```python
from build123d import *

# Parameters (mm, degrees)
SKETCH1_W           = 20
SKETCH1_H           = 30
BOSS_EXTRUDE1_DEPTH = 10
BOSS_EXTRUDE2_DEPTH = 10
SKETCH4_R           = 8.55
BOSS_EXTRUDE3_DEPTH = 10
FILLET1_R           = 5
BOSS_EXTRUDE4_DEPTH = 10
SKETCH6_R           = 1.25
CUT_EXTRUDE1_DEPTH  = 10


with BuildPart() as part:
    # Sketch1 → Boss-Extrude1 (new body)
    with BuildSketch(Plane(origin=(0, 0, 0), x_dir=(1, 0, 0), z_dir=(0, 1, 0))):
        with Locations((10, -15)):
            Rectangle(SKETCH1_W, SKETCH1_H)
    extrude(amount=BOSS_EXTRUDE1_DEPTH)

    # Sketch2 → Boss-Extrude2 (add)
    with BuildSketch(Plane(origin=(0, 10, 0), x_dir=(1, 0, 0), z_dir=(0, 1, 0))):
        Polygon((0, 0), (0, -10), (10, -10), (10, -30), (20, -30), (20, 0), align=None)
    extrude(amount=BOSS_EXTRUDE2_DEPTH)

    # Sketch4 → Boss-Extrude3 (add)
    with BuildSketch(Plane(origin=(0, 10, 0), x_dir=(1, 0, 0), z_dir=(0, 1, 0))):
        with BuildLine():
            Line((0, 0), (-17.51372228, 3.319944561))
            ThreePointArc((-17.51372228, 3.319944561), (-33.173842605, -6.829452566), (-23.846362973, -22.992612973))
            Line((-23.846362973, -22.992612973), (0, -30))
            Line((0, -30), (0, 0))
        make_face()
        with Locations(Location((-20, -10, 0), (0, 0, 270))):
            Circle(SKETCH4_R, mode=Mode.SUBTRACT)
    extrude(amount=-BOSS_EXTRUDE3_DEPTH)

    # Fillet1
    fillet1_edges = [part.edges().sort_by_distance(p)[0] for p in [
        (0, 10, 5),
        (20, 0, 15),
        (20, 10, 0),
        (20, 10, 30),
    ]]
    fillet(fillet1_edges, radius=FILLET1_R)

    # Sketch5 → Boss-Extrude4 (add)
    with BuildSketch(Plane(origin=(0, 20, 0), x_dir=(1, 0, 0), z_dir=(0, 1, 0))):
        with BuildLine():
            Line((10, -30), (15, -30))
            ThreePointArc((15, -30), (18.535533906, -28.535533906), (20, -25))
            Line((20, -25), (20, -5))
            ThreePointArc((20, -5), (18.535533906, -1.464466094), (15, 0))
            Line((15, 0), (0, 0))
            Line((0, 0), (0, -10))
            Line((0, -10), (10, -10))
            Line((10, -10), (10, -30))
        make_face()
    extrude(amount=BOSS_EXTRUDE4_DEPTH)

    # Sketch6 → Cut-Extrude1 (cut)
    with BuildSketch(Plane.ZY.offset(-10)):
        with Locations((20, 20)):
            Circle(SKETCH6_R)
    extrude(amount=-CUT_EXTRUDE1_DEPTH, mode=Mode.SUBTRACT)


solid = part.part
```
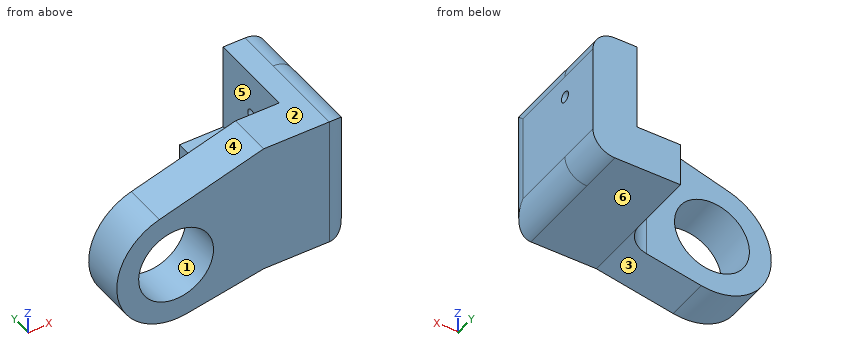
Verification items for the finished model (mm, model axes). Face numbers are marked on the shaded views. A direction names the side the tool comes from. Round coordinates to 2 decimals unless told otherwise and drop trailing zeros. Write each loop counter-clockwise with the first axis right and the second up, starting at its lowest first coordinate (ties: lowest second). Pieces come first, ordered by that corner, then holes.
1. Section check C-C on z = 16. Enter the section's corners in (x, y), plus the area to 3 significant figures.
2. Section check A-A on y = 15.75. Enter the section's corners in (x, z), plus the area to 3 significant figures.
3. Gauge pin test, flat ends, axial feed: P1, Ø6, axis at x = -16, z = 17.5, coming from the +Y side; P2, Ø10, axis at y = 18.5, z = 20, coming from the -X side; P3, Ø11, axis at y = 20, z = 5, coming from the -X side. Record the tip position at first contact, or that the pin passes through.
4. Section check D-D on y = 7. Enter the section's corners in (x, z).
5. Section check B-B on x = -20. Enter the section's corners in (y, z).
6. Access from +Z, -Z, +X, -X, +Y, -Y to the whole of each face (thin tool, end or side, straight path). Record for the marked faces 4, 5 and 6.
7. Scan lines: L1, parallel to Z at x = 0.5, y = 11; L2, parallel to X at y = 20.25, z = 16; L3, parallel to Y at x = 13, z = 21. Record each from-to range of solid material in increasing order.
8. Draft check along X on the marked faces 1, 2 and 3. Enter one of: +X half, -X half, draft (parallel to the pull), parting line (faces both ways), or undercut.
Answer:
1. outline: (-32.15, 0) - (-26.09, 0) - (-26.09, 10) - (-32.15, 10) - close; (-13.91, 0) - (15, 0) arc R5 ccw to (20, 5) - (20, 30) - (10, 30) - (10, 10) - (-13.91, 10) - close
1. area: 594 mm2
2. outline: (0, 0) - (15, 0) arc R5 ccw to (20, 5) - (20, 25) arc R5 ccw to (15, 30) - (10, 30) - (10, 10) - (0, 10) - close
2. area: 389 mm2
3. P1: stops at y = 10
3. P2: stops at x = 10
3. P3: stops at x = -0.03
4. outline: (-23.85, 22.99) arc R13.55 ccw to (-17.51, -3.32) - (0, 0) - (15, 0) arc R5 ccw to (20, 5) - (20, 25) arc R5 ccw to (15, 30) - (0, 30) - close; hole circle Ø17.1 at (-20, 10)
5. outline: (0, -3.55) - (10, -3.55) - (10, 1.45) - (0, 1.45) - close; (0, 18.55) - (10, 18.55) - (10, 24.12) - (0, 24.12) - close
6. face 4: +Z, -X, +Y, -Y
6. face 5: +Z, -X, +Y
6. face 6: -Z, +X, +Y, -Y
7. L1: z = 0 to 10
7. L2: x = 10 to 20
7. L3: y = 0 to 19.25, 20.75 to 30
8. face 1: undercut
8. face 2: draft
8. face 3: +X half
